The model under review builds one solid part; all positions refer to its coordinate system, in mm. Face numbers are marked on the shaded views. Give positions to 0.01 mm unless a question says otherwise; leave off trailing zeros. Loops run counter-clockwise (first coordinate to the right, second up) from the corner with the lowest first, then second, coordinate; pieces in that order, holes last. Notation, with made-up numbers: M 51,55 L 93,55 A15 ccw 93,61 Z; hole C 24.25,64 d4. An arc over 180 degrees is marked long. Put each result on its own line as item: value. Start each with the question number.
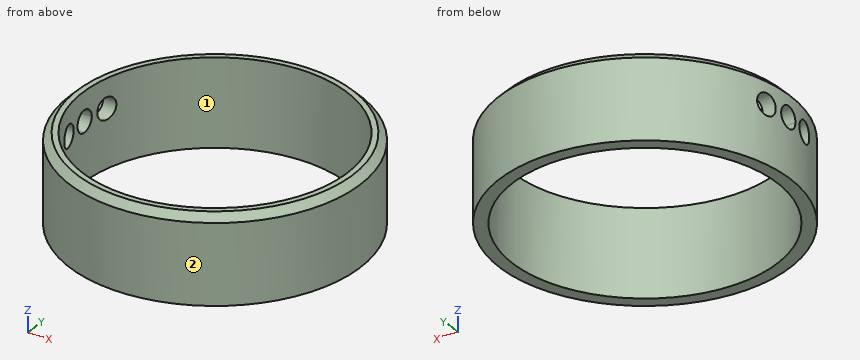
```python
from build123d import *

# Parameters (mm, degrees)
F0_R     = 10
F0_R_2   = 9.1
F1_DEPTH = 6
F2_R     = 0.75
F3_DEPTH = 25
F4_SIZE  = 0.5


with BuildPart() as f1:
    # F0 (on Top) → F1 (new body)
    with BuildSketch(Plane.XY):
        Circle(F0_R)
        Circle(F0_R_2, mode=Mode.SUBTRACT)
    extrude(amount=F1_DEPTH)

    # F2 (on Right) → F3 (cut)
    with BuildSketch(Plane.YZ):
        with BuildLine():
            ThreePointArc((2.75, 4), (2, 4.75), (1.25, 4))
            ThreePointArc((1.25, 4), (2, 3.25), (2.75, 4))
        make_face()
        with BuildLine():
            Line((0, 4), (0, 3.25))
            ThreePointArc((0, 3.25), (0.53033, 3.46967), (0.75, 4))
            Line((0.75, 4), (0, 4))
        make_face()
        with BuildLine():
            Line((-0.75, 4), (0, 4))
            Line((0, 4), (0.75, 4))
            ThreePointArc((0.75, 4), (0, 4.75), (-0.75, 4))
        make_face()
        with BuildLine():
            ThreePointArc((-0.75, 4), (-0.53033, 3.46967), (0, 3.25))
            Line((0, 3.25), (0, 4))
            Line((0, 4), (-0.75, 4))
        make_face()
        with Locations((-2, 4)):
            Circle(F2_R)
    extrude(amount=-F3_DEPTH, mode=Mode.SUBTRACT)

    # F4
    f4_edges = [f1.edges().sort_by_distance(p)[0] for p in [
        (-10, 0, 6),
    ]]
    chamfer(f4_edges, length=F4_SIZE)


solid = f1.part
```
Item 1: Consider section C-C, the plane z = 5.75. Write out the cut boundary in (x, y).
Item 2: Consider section A-A, the plane x = 0. Write out the cut boundary in (y, z), plus the area to 4 significant figures.
Item 3: Clearance check with flat-ended pins moving along their axes: pin 1 Ø0.9 at (y, z) = (2, 4) entering from -X; pin 2 Ø1.2 at (y, z) = (-2, 4) entering from -X. State where each tip first meets the part, or that it passes through.
Item 4: Consider section B-B, the plane z = 4.5. Write out the cut boundary in (x, y), plus the area to 3 significant figures.
Item 5: Draft analysis for pull direction Y (two halves, no side actions). For the marked faces 1 and 2, state which applies: +Y half, -Y half, draft (parallel to the pull), parting line (faces both ways), or undercut.
Item 6: Consider section D-D, the plane y = -2. Give the number of separate pieces and of enclosed holes in the cut face, plus the area to 3 significant figures.
Item 7: To check wall thickness, follow L1, parallel to Y at x = 0, z = 2.5; L2, parallel to Z at x = -9.25, y = 2; L3, parallel to Y at x = -8.95, z = 4. State the ranges of each line that lie inside material, in increasing order. Write a range as [from, to].
Report:
1. outline: C 0,0 d19.5; hole C 0,0 d18.2
2. outline: M -10,0 L -9.1,0 L -9.1,6 L -9.5,6 L -10,5.5 Z; M 9.1,0 L 10,0 L 10,5.5 L 9.5,6 L 9.1,6 Z
2. area: 10.55 mm²
3. pin 1: x = 8.76
3. pin 2: x = 8.72
4. outline: M -9.98,-0.56 A10 ccw -9.9,-1.44 L -8.99,-1.44 A9.1 cw -9.08,-0.56 Z; M -9.98,0.56 L -9.08,0.56 A9.1 cw -8.99,1.44 L -9.9,1.44 A10 ccw Z; M -9.67,-2.56 A10 ccw long -9.67,2.56 L -8.73,2.56 A9.1 cw long -8.73,-2.56 Z
4. area: 50.9 mm²
5. face 1: undercut
5. face 2: parting line
6. separate pieces: 3
6. enclosed holes: 0
6. area: 9.41 mm²
7. L1: [-10, -9.1], [9.1, 10]
7. L2: [0, 3.25], [4.75, 6]
7. L3: [-4.46, -2.75], [2.75, 4.46]
